Here's how the part is built. I have some questions about the finished solid (model axes, mm). Coordinates: 2 decimals unless noted, no trailing zeros. Order: outer loops, then holes, each group sorted by start corner. A loop starts at its lowest first (then second) coordinate and runs counter-clockwise, first axis right, second up.
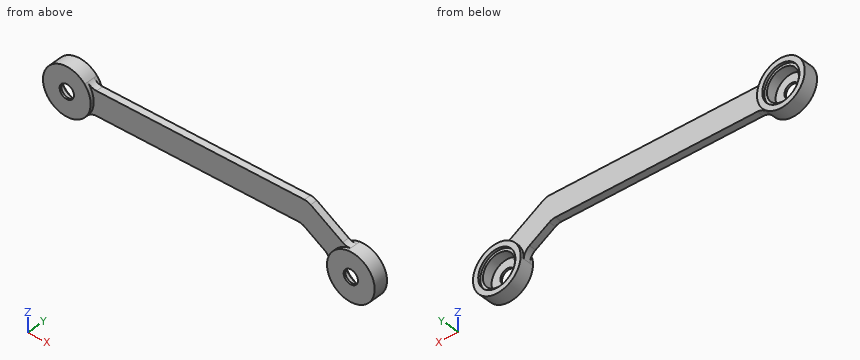
```python
from build123d import *
from build123d.topology import SkipClean

# Parameters (mm, degrees)
SKETCH1_R           = 7.8
SKETCH1_R_2         = 3
BOSS_EXTRUDE2_DEPTH = 3
SKETCH2_R           = 7.8
CUT_EXTRUDE1_DEPTH  = 1
SKETCH3_R           = 6.7
CUT_EXTRUDE2_DEPTH  = 5.2
CUT_EXTRUDE4_DEPTH  = 1.5
CUT_EXTRUDE5_START  = -1.5
CUT_EXTRUDE5_DEPTH  = 1.5


with BuildPart() as part:
    # Sketch1 → Boss-Extrude2 (new, symmetric)
    # profile 1 of 3: a face of its own
    with BuildSketch(Plane(origin=(0, 0, 0), x_dir=(1, 0, 0), z_dir=(0, 1, 0))):
        with BuildLine():
            ThreePointArc((7.453559925, 6.666666667), (9.139098435, 5.435645354), (11.180339887, 5))
            Line((11.180339887, 5), (95.787507262, 5))
            ThreePointArc((95.787507262, 5), (97.157669446, 5.191397751), (98.422933246, 5.750937765))
            Line((98.422933246, 5.750937765), (106.744136599, 10.912056694))
            ThreePointArc((106.744136599, 10.912056694), (108.435692963, 12.655680094), (109.105807076, 14.990745953))
            ThreePointArc((109.105807076, 14.990745953), (126.766700664, 21.070412832), (117.680813085, 4.751216817))
            ThreePointArc((117.680813085, 4.751216817), (115.946610906, 4.695717028), (114.335793643, 4.050887461))
            Line((114.335793643, 4.050887461), (100.953895224, -4.249062235))
            ThreePointArc((100.953895224, -4.249062235), (99.688631423, -4.808602249), (98.318469239, -5))
            Line((98.318469239, -5), (11.180339887, -5))
            ThreePointArc((11.180339887, -5), (9.139098435, -5.435645354), (7.453559925, -6.666666667))
            ThreePointArc((7.453559925, -6.666666667), (-10, 0), (7.453559925, 6.666666667))
        make_face()
        with Locations((119.1, 14.65)):
            Circle(SKETCH1_R, mode=Mode.SUBTRACT)
        Circle(SKETCH1_R, mode=Mode.SUBTRACT)
    # profile 2 of 3: a face of its own
    with BuildSketch(Plane(origin=(0, 0, 0), x_dir=(1, 0, 0), z_dir=(0, 1, 0))):
        Circle(SKETCH1_R)
        with Locations(Location((0, 0, 0), (0, 0, 270))):
            Circle(SKETCH1_R_2, mode=Mode.SUBTRACT)
    # profile 3 of 3: a face of its own
    with BuildSketch(Plane(origin=(0, 0, 0), x_dir=(1, 0, 0), z_dir=(0, 1, 0))):
        with Locations((119.1, 14.65)):
            Circle(SKETCH1_R)
        with Locations(Location((119.1, 14.65, 0), (0, 0, 270))):
            Circle(SKETCH1_R_2, mode=Mode.SUBTRACT)
    extrude(amount=BOSS_EXTRUDE2_DEPTH, both=True)

    # Sketch2 → Cut-Extrude1 (cut)
    with BuildSketch(Plane(origin=(0, 3, 0), x_dir=(1, 0, 0), z_dir=(0, 1, 0))):
        with Locations(Location((119.1, 14.65, 0), (0, 0, 270))):
            Circle(SKETCH2_R)
        with Locations(Location((0, 0, 0), (0, 0, 270))):
            Circle(SKETCH2_R)
    extrude(amount=-CUT_EXTRUDE1_DEPTH, mode=Mode.SUBTRACT)

    # Sketch3 → Cut-Extrude2 (cut)
    with BuildSketch(Plane(origin=(0, 3, 0), x_dir=(1, 0, 0), z_dir=(0, 1, 0))):
        with Locations(Location((0, 0, 0), (0, 0, 270))):
            Circle(SKETCH3_R)
        with Locations(Location((119.1, 14.65, 0), (0, 0, 270))):
            Circle(SKETCH3_R)
    extrude(amount=-CUT_EXTRUDE2_DEPTH, mode=Mode.SUBTRACT)

    # Sketch4 → Cut-Extrude4 (cut)
    with BuildSketch(Plane(origin=(0, 3, 0), x_dir=(1, 0, 0), z_dir=(0, 1, 0))):
        with BuildLine():
            Line((106.744136599, 10.912056694), (98.422933246, 5.750937765))
            ThreePointArc((98.422933246, 5.750937765), (97.157669446, 5.191397751), (95.787507262, 5))
            Line((95.787507262, 5), (11.180339887, 5))
            ThreePointArc((11.180339887, 5), (9.139098435, 5.435645354), (7.453559925, 6.666666667))
            ThreePointArc((7.453559925, 6.666666667), (9.34172359, 3.568220898), (10, 0))
            ThreePointArc((10, 0), (9.34172359, -3.568220898), (7.453559925, -6.666666667))
            ThreePointArc((7.453559925, -6.666666667), (9.139098435, -5.435645354), (11.180339887, -5))
            Line((11.180339887, -5), (98.318469239, -5))
            ThreePointArc((98.318469239, -5), (99.688631423, -4.808602249), (100.953895224, -4.249062235))
            Line((100.953895224, -4.249062235), (114.335793643, 4.050887461))
            ThreePointArc((114.335793643, 4.050887461), (115.946610906, 4.695717028), (117.680813085, 4.751216817))
            ThreePointArc((117.680813085, 4.751216817), (111.433299336, 8.229587168), (109.105807076, 14.990745953))
            ThreePointArc((109.105807076, 14.990745953), (108.435692963, 12.655680094), (106.744136599, 10.912056694))
        make_face()
    extrude(amount=-CUT_EXTRUDE4_DEPTH, mode=Mode.SUBTRACT)

    # Sketch5 → Cut-Extrude5 (cut)
    with SkipClean():  # the faces are left unmerged after this step: merging them gives an invalid solid
        with BuildSketch(Plane.XZ.offset(3).offset(CUT_EXTRUDE5_START)):
            with BuildLine():
                ThreePointArc((7.453559925, 6.666666667), (9.34172359, 3.568220898), (10, 0))
                ThreePointArc((10, 0), (9.34172359, -3.568220898), (7.453559925, -6.666666667))
                ThreePointArc((7.453559925, -6.666666667), (9.139098435, -5.435645354), (11.180339887, -5))
                Line((11.180339887, -5), (95.787507262, -5))
                ThreePointArc((95.787507262, -5), (97.157669446, -5.191397751), (98.422933246, -5.750937765))
                Line((98.422933246, -5.750937765), (106.744136599, -10.912056694))
                ThreePointArc((106.744136599, -10.912056694), (108.435692963, -12.655680094), (109.105807076, -14.990745953))
                ThreePointArc((109.105807076, -14.990745953), (111.433299336, -8.229587168), (117.680813085, -4.751216817))
                ThreePointArc((117.680813085, -4.751216817), (115.946610906, -4.695717028), (114.335793643, -4.050887461))
                Line((114.335793643, -4.050887461), (100.953895224, 4.249062235))
                ThreePointArc((100.953895224, 4.249062235), (99.688631423, 4.808602249), (98.318469239, 5))
                Line((98.318469239, 5), (11.180339887, 5))
                ThreePointArc((11.180339887, 5), (9.139098435, 5.435645354), (7.453559925, 6.666666667))
            make_face()
        extrude(amount=CUT_EXTRUDE5_DEPTH, mode=Mode.SUBTRACT)


solid = part.part
```
Q1. I need wall thicknesses on L1, parallel to Z at x = 0, y = 2.75; L2, parallel to X at y = -0.35, z = -14.65; L3, parallel to X at y = -2.1, z = -7.5. Which ranges of each line are inside material? Lowest first, please.
Q2. If we section it at B-B on y = 0.5: Write out the boundary of the cut face in (x, z), then the cut area to 3 significant figures.
Q3. If we section it at A-A on x = 119.1: Write out the boundary of the cut face in (y, z).
Q4. Will these pins go through, and if not, where does the flat tip stop? pin 1 (1.5 mm diameter, centred on x = 56, y = -0.5, fed in from -Z); pin 2 (4 mm diameter, centred on x = 30.5, z = -3, fed in from +Y); pin 3 (9.5 mm diameter, centred on x = 119.1, z = -14.65, fed in from +Y).
Q5. If we section it at C-C on x = 54.5: Write out the boundary of the cut face in (y, z).
Reply:
1. L1: z = -10 to -7.8, 7.8 to 10
1. L2: x = 109.08 to 112.4, 125.8 to 129.1
1. L3: x = -6.61 to 6.61, 112.11 to 126.09
2. outline: (7.45, -6.67) arc R5 cw to (11.18, -5) - (95.79, -5) arc R5 cw to (98.42, -5.75) - (106.74, -10.91) arc R5 cw to (109.11, -14.99) arc R10 ccw (long way) to (117.68, -4.75) arc R5 cw to (114.34, -4.05) - (100.95, 4.25) arc R5 ccw to (98.32, 5) - (11.18, 5) arc R5 cw to (7.45, 6.67) arc R10 ccw (long way) to start; hole circle Ø13.4 at (0, 0); hole circle Ø13.4 at (119.1, -14.65)
2. area: 1,390 mm2
3. outline: (-3, -24.65) - (3, -24.65) - (3, -22.45) - (2, -22.45) - (2, -21.35) - (-2.2, -21.35) - (-2.2, -17.65) - (-3, -17.65) - close; (-3, -11.65) - (-2.2, -11.65) - (-2.2, -7.95) - (2, -7.95) - (2, -6.85) - (3, -6.85) - (3, -4.65) - (-3, -4.65) - close
4. pin 1: stops at z = -5
4. pin 2: stops at y = 1.5
4. pin 3: stops at y = -2.2
5. outline: (-1.5, -5) - (1.5, -5) - (1.5, 5) - (-1.5, 5) - close
